```python
from build123d import *

# Parameters (mm, degrees)
SKETCH1_R           = 8.45
BOSS_EXTRUDE1_DEPTH = 7
SKETCH2_R           = 10
BOSS_EXTRUDE2_DEPTH = 4.5
SKETCH3_R           = 8.45
BOSS_EXTRUDE3_DEPTH = 6
SKETCH4_R           = 8.45
BOSS_EXTRUDE4_DEPTH = 1
SKETCH5_W           = 9
SKETCH5_H           = 6
BOSS_EXTRUDE5_DEPTH = 4
SKETCH6_R           = 1.5
CUT_EXTRUDE1_DEPTH  = 8
CUT_EXTRUDE4_DEPTH  = 10
CHAMFER1_SIZE       = 1


with BuildPart() as part:
    # Sketch1 → Boss-Extrude1 (new body)
    with BuildSketch(Plane(origin=(0, 0, 0), x_dir=(1, 0, 0), z_dir=(0, 1, 0))):
        Circle(SKETCH1_R)
    extrude(amount=BOSS_EXTRUDE1_DEPTH)

    # Sketch2 → Boss-Extrude2 (add)
    with BuildSketch(Plane(origin=(0, 7, 0), x_dir=(1, 0, 0), z_dir=(0, 1, 0))):
        Circle(SKETCH2_R)
    extrude(amount=BOSS_EXTRUDE2_DEPTH)

    # Sketch3 → Boss-Extrude3 (add)
    with BuildSketch(Plane(origin=(0, 11.5, 0), x_dir=(1, 0, 0), z_dir=(0, 1, 0))):
        with Locations((0, 1.5)):
            Circle(SKETCH3_R)
    extrude(amount=BOSS_EXTRUDE3_DEPTH)

    # Sketch4 → Boss-Extrude4 (add)
    with BuildSketch(Plane(origin=(0, 11.5, 0), x_dir=(1, 0, 0), z_dir=(0, 1, 0))):
        with BuildLine():
            ThreePointArc((9.971835338, 0.75), (0, 10), (-9.971835338, 0.75))
            ThreePointArc((-9.971835338, 0.75), (0, -8.5), (9.971835338, 0.75))
        make_face()
        with Locations((0, 1.5)):
            Circle(SKETCH4_R, mode=Mode.SUBTRACT)
    extrude(amount=BOSS_EXTRUDE4_DEPTH)

    # Sketch5 → Boss-Extrude5 (add)
    with BuildSketch(Plane(origin=(0, 17.5, 0), x_dir=(1, 0, 0), z_dir=(0, 1, 0))):
        Rectangle(SKETCH5_W, SKETCH5_H)
    extrude(amount=BOSS_EXTRUDE5_DEPTH)

    # Sketch6 → Cut-Extrude1 (cut)
    with BuildSketch(Plane(origin=(0, 21.5, 0), x_dir=(1, 0, 0), z_dir=(0, 1, 0))):
        Circle(SKETCH6_R)
    extrude(amount=-CUT_EXTRUDE1_DEPTH, mode=Mode.SUBTRACT)

    # Sketch9 → Cut-Extrude4 (cut)
    with BuildSketch(Plane(origin=(0, 0, 0), x_dir=(-1, 0, 0), z_dir=(0, -1, 0))):
        with BuildLine():
            Line((1.319090596, -1.15), (-1.319090596, -1.15))
            ThreePointArc((-1.319090596, -1.15), (0, 1.75), (1.319090596, -1.15))
        make_face()
    extrude(amount=-CUT_EXTRUDE4_DEPTH, mode=Mode.SUBTRACT)

    # Chamfer1
    chamfer1_edges = [part.edges().sort_by_distance(p)[0] for p in [
        (0, 0, -1.75),
        (0, 0, 1.15),
    ]]
    chamfer(chamfer1_edges, length=CHAMFER1_SIZE)


solid = part.part
```
Part model, mm, in its own coordinate system. A direction names the side the tool comes from. Round coordinates to 2 decimals unless told otherwise and drop trailing zeros. Loops run counter-clockwise (first coordinate to the right, second up) from the corner with the lowest first, then second, coordinate; pieces in that order, holes last.
1. Slice it at B-B (x = 0). Give the cut face in (y, z), and give its area (3 significant figures).
Solutions:
outline: (0, -8.45) - (7, -8.45) - (7, -10) - (12.5, -10) - (12.5, -9.95) - (17.5, -9.95) - (17.5, -3) - (21.5, -3) - (21.5, -1.5) - (13.5, -1.5) - (13.5, 1.5) - (21.5, 1.5) - (21.5, 3) - (17.5, 3) - (17.5, 6.95) - (12.5, 6.95) - (12.5, 8.5) - (11.5, 8.5) - (11.5, 10) - (7, 10) - (7, 8.45) - (0, 8.45) - (0, 2.15) - (1, 1.15) - (10, 1.15) - (10, -1.75) - (1, -1.75) - (0, -2.75) - close
area: 281 mm2
2. Drill centre lines: line 1 along Z through (x, y) = (0, 17.25); line 2 along X through (y, z) = (8, 0); line 3 along X through (y, z) = (5, 0). Where is each one in solid material? Low to high.
Solutions:
line 1: z = -9.95 to -1.5, 1.5 to 6.95
line 2: x = -10 to -1.75, 1.75 to 10
line 3: x = -8.45 to -1.75, 1.75 to 8.45
3. Slice it at D-D (y = 8.5). Give the cut face in (x, z).
Solutions:
outline: circle Ø20 at (0, 0); hole (-1.32, 1.15) arc R1.75 ccw (long way) to (1.32, 1.15) - close
4. Flat gauge pins, fed straight in: pin 1 (10 mm diameter, centred on x = 7.5, y = 9, fed in from +Z); pin 2 (1.4 mm diameter, centred on x = -0.5, z = -0.5, fed in from -Y); pin 3 (4 mm diameter, centred on y = 16.5, z = -1.5, fed in from -X). Where does each tip first touch, or does it go through?
Solutions:
pin 1: stops at z = 9.68
pin 2: stops at y = 10
pin 3: stops at x = -8.45
5. Two-plate mould, pull along X, no slides. Class faces 1 (the face through (8.06, 3.45, -2.54)), 2 (the face through (0.07, 0.84, -1.91)), 3 (the face through (0, 19, 3)): pulls with the +X half, pulls with the -X half, needs draft (parallel to the pull), parting line crosses it, or undercut.
Solutions:
face 1: parting line crosses it
face 2: undercut
face 3: needs draft
6. Slice it at A-A (y = 19). Give the cut face in (x, z).
Solutions:
outline: (-4.5, -3) - (4.5, -3) - (4.5, 3) - (-4.5, 3) - close; hole circle Ø3 at (0, 0)
7. 3-axis set-ups, long thin cutter, end or side, ignore diameter. For faces 4 (the face through (4.5, 19, 0)), 5 (the face through (0, 19, -3)), 6 (the face through (0, 5, 1.15)), 7 (the face through (8.06, 14.96, -4.04)), 8 (the face through (-0.2, 12, 8.5)): which of +Z, -Z, +X, -X, +Y, -Y reach the whole face in a straight line?
Solutions:
face 4: +Z, -Z, +X, +Y
face 5: -Z, +X, -X, +Y
face 6: -Y
face 7: +Y
face 8: +Z, +Y
8. Slice it at C-C (z = 6.5). Give the cut face in (x, y), and give its area (3 significant figures).
Solutions:
outline: (-7.6, 7) - (-5.4, 7) - (-5.4, 0) - (5.4, 0) - (5.4, 7) - (7.6, 7) - (7.6, 11.5) - (6, 11.5) - (6, 12.5) - (2.72, 12.5) - (2.72, 17.5) - (-2.72, 17.5) - (-2.72, 12.5) - (-6, 12.5) - (-6, 11.5) - (-7.6, 11.5) - close
area: 183 mm2
